from build123d import *

# Parameters (mm, degrees)
F0_W     = 127
F0_H     = 76.2
F1_DEPTH = 25.4
F3_DEPTH = 25.4
F5_DEPTH = 25.4
F7_DEPTH = 94.22763


# Not quite as in the source:
# - a feature names something its author has since deleted; it is built from what else it names


with BuildPart() as f1:
    # F0 (on Top) → F1 (new body)
    with BuildSketch(Plane.XY):
        with Locations((4.9490761012, -17.8116933908)):
            Rectangle(F0_W, F0_H)
    extrude(amount=F1_DEPTH)

    # F2 (on face) → F3 (cut)
    with BuildSketch(Plane.XY.offset(25.4)):
        with BuildLine():
            Line((43.0490761012, -55.9116933908), (68.4490761012, -55.9116933908))
            Line((68.4490761012, -55.9116933908), (68.4490761012, -17.8116933908))
            Line((68.4490761012, -17.8116933908), (68.4490761012, 20.2883066092))
            Line((68.4490761012, 20.2883066092), (43.0490761012, 20.2883066092))
            ThreePointArc((43.0490761012, 20.2883066092), (65.0746365727, -17.8116933908), (43.0490761012, -55.9116933908))
        make_face()
    extrude(amount=-F3_DEPTH, mode=Mode.SUBTRACT)

    # F4 (on face) → F5 (cut)
    with BuildSketch(Plane.XY.offset(25.4)):
        with BuildLine():
            ThreePointArc((8.3779023105, -27.1882303593), (20.0063433992, -27.7934270204), (26.0023336343, -17.8116933908))
            ThreePointArc((26.0023336343, -17.8116933908), (20.0437900528, -7.8499724051), (8.4485028496, -8.387969882))
            ThreePointArc((8.4485028496, -8.387969882), (9.7226855998, -12.9646479051), (10.1520907288, -17.695941031))
            ThreePointArc((10.1520907288, -17.695941031), (9.7047360462, -22.5242766975), (8.3779023105, -27.1882303593))
        make_face()
        with BuildLine():
            ThreePointArc((10.1520907288, -17.695941031), (9.7226855998, -12.9646479051), (8.4485028496, -8.387969882))
            ThreePointArc((8.4485028496, -8.387969882), (3.3894837429, -17.7692345704), (8.3779023105, -27.1882303593))
            ThreePointArc((8.3779023105, -27.1882303593), (9.7047360462, -22.5242766975), (10.1520907288, -17.695941031))
        make_face()
        with BuildLine():
            ThreePointArc((8.3779023105, -27.1882303593), (3.3894837429, -17.7692345704), (8.4485028496, -8.387969882))
            ThreePointArc((8.4485028496, -8.387969882), (-11.8448406538, 8.2326764046), (-36.4052897795, -0.9787302349))
            ThreePointArc((-36.4052897795, -0.9787302349), (-28.6441463529, -5.3094690784), (-25.5636865376, -13.646219857))
            ThreePointArc((-25.5636865376, -13.646219857), (-30.2938818163, -23.5920338801), (-40.9942057814, -26.1991454999))
            ThreePointArc((-40.9942057814, -26.1991454999), (-16.6542659577, -43.9706572732), (8.3779023105, -27.1882303593))
        make_face()
        with BuildLine():
            ThreePointArc((-40.9942057814, -26.1991454999), (-41.9833758583, -12.9914737388), (-36.4052897795, -0.9787302349))
            ThreePointArc((-36.4052897795, -0.9787302349), (-50.9990660995, -11.3510469345), (-40.9942057814, -26.1991454999))
        make_face()
        with BuildLine():
            ThreePointArc((-25.5636865376, -13.646219857), (-28.6441463529, -5.3094690784), (-36.4052897795, -0.9787302349))
            ThreePointArc((-36.4052897795, -0.9787302349), (-41.9833758583, -12.9914737388), (-40.9942057814, -26.1991454999))
            ThreePointArc((-40.9942057814, -26.1991454999), (-30.2938818163, -23.5920338801), (-25.5636865376, -13.646219857))
        make_face()
    extrude(amount=-F5_DEPTH, mode=Mode.SUBTRACT)

    # F6 (on face) → F7 (cut)
    with BuildSketch(Plane.XZ.offset(55.9116933908)):
        with BuildLine():
            Line((43.0490761012, 25.4), (-58.5509238988, 25.4))
            ThreePointArc((-58.5509238988, 25.4), (-7.7509238988, 12.7), (43.0490761012, 25.4))
        make_face()
    extrude(amount=-F7_DEPTH, mode=Mode.SUBTRACT)


solid = f1.part
The model under review builds one solid part; all positions refer to its coordinate system, in mm. A direction names the side the tool comes from. Round coordinates to 2 decimals unless told otherwise and drop trailing zeros. Order: outer loops, then holes, each group sorted by start corner. A loop starts at its lowest first (then second) coordinate and runs counter-clockwise, first axis right, second up. Notation, with made-up numbers: (13.5, 9) -> (21.5, 9) arc R25 ccw to (21.5, 46) -> close; hole circle Ø4 at (86.25, -1.5). An arc over 180 degrees is marked (long way). Return JSON: item names as keys, results as strings.
1. For faces 5 (the face through (-11.466, 8.167, 6.561)), 6 (the face through (51, -17, 25.4)), list the 3-axis set-ups (+Z, -Z, +X, -X, +Y, -Y) from which the entire face can be reached by the end or side of a thin tool; tool diameter is ignored.
Answer block:
{"face 5": "+Z, -Z", "face 6": "+Z, +X, -X, +Y, -Y"}
2. Insertion check: P1, Ø3, axis at x = 32.5, y = 2.5, coming from the +Z side; P2, Ø8, axis at y = -42.5, z = 21.5, coming from the +X side; P3, Ø3, axis at x = -38, y = 3.5, coming from the +Z side. Each pin has a flat end and moves straight along its axis. Give the tip position at first contact, or say it passes through.
Answer block:
{"P1": "stops at z = 21.1", "P2": "stops at x = 59.9", "P3": "stops at z = 17.47"}
3. Take a section at B-B (x = 21). Write out the cut boundary in (y, z).
Answer block:
{"outline": "(-55.91, 0) -> (-27.2, 0) -> (-27.2, 16.6) -> (-55.91, 16.6) -> close; (-8.43, 0) -> (20.29, 0) -> (20.29, 16.6) -> (-8.43, 16.6) -> close"}
4. For L1, parallel to X at y = -16, z = 4; L2, parallel to Y at x = -49.5, z = 4.5; L3, parallel to X at y = -25.5, z = 20.5, list the stretches that pass through material, from the lowest coordinate up. Write a range as [from, to].
Answer block:
{"L1": "x = [-58.55, -50.99], [25.86, 65.04]", "L2": "y = [-55.91, -20.04], [-7.26, 20.29]", "L3": "x = [-58.55, -48.04], [32.54, 64.4]"}
5. Take a section at C-C (z = 8.75). Write out the cut boundary in (x, y), then the cut area to 3 significant figures.
Answer block:
{"outline": "(-58.55, -55.91) -> (43.05, -55.91) arc R43.97 ccw to (43.05, 20.29) -> (-58.55, 20.29) -> close; hole (-40.99, -26.2) arc R26.28 ccw to (8.38, -27.19) arc R11.31 ccw (long way) to (8.45, -8.39) arc R26.28 ccw to (-36.41, -0.98) arc R12.82 ccw to start", "area": "6,260 mm²"}
6. The part is to be moulded in two halves that separate along Y. For faces 1 (the face through (65.07, -17.17, 12.88)), 2 (the face through (-50.946, -11.079, 11.069)), 3 (the face through (-17.103, -43.958, 7.105)), 4 (the face through (-58.551, -18, 13)), say which applies: +Y half, -Y half, draft (parallel to the pull), parting line (faces both ways), or undercut.
Answer block:
{"face 1": "parting line", "face 2": "undercut", "face 3": "undercut", "face 4": "draft"}
7. Take a section at D-D (z = 19.75). Write out the cut boundary in (x, y), then the cut area to 3 significant figures.
Answer block:
{"outline": "(-58.55, -55.91) -> (-46.12, -55.91) -> (-46.12, -23.87) arc R12.82 cw to (-46.12, -3.42) -> (-46.12, 20.29) -> (-58.55, 20.29) -> close; (30.62, -55.91) -> (43.05, -55.91) arc R43.97 ccw to (43.05, 20.29) -> (30.62, 20.29) -> close", "area": "3,010 mm²"}
8. Take a section at A-A (y = -21). Write out the cut boundary in (x, z), then the cut area to 3 significant figures.
Answer block:
{"outline": "(-58.55, 0) -> (-48.89, 0) -> (-48.89, 20.85) arc R107.95 cw to (-58.55, 25.4) -> close; (25.54, 0) -> (64.96, 0) -> (64.96, 25.4) -> (43.05, 25.4) arc R107.95 cw to (25.54, 17.96) -> close", "area": "1,150 mm²"}
